Input: dimensioned drawing with shaded views. Units: mm. Origin: part minimum x, y, z. Give positions to 0.01 mm unless a question says otherwise; leave off trailing zeros. Write each loop counter-clockwise with the first axis right and the second up, starting at its lowest first coordinate (ties: lowest second). Pieces come first, ordered by that corner, then holes. Notation, with made-up numbers: (-28.75, 77) -> (1.25, 77) arc R20 cw to (1.25, 109) -> close; hole circle Ø3 at (74.5, -36.75). An arc over 180 degrees is marked (long way). Return JSON: item names as keys, results as strings. Group by question number.
Item 1: Section B-B, the plane z = 0.7. Return loops of the section in (x, y) (1 decimal).
Item 2: Line query: line 1 (Y direction, x = 203.2, z = 1.5); line 2 (Y direction, x = 109.5, z = 1.3) (1 decimal); line 3 (Y direction, x = 114, z = 0.15) (1 decimal). Output: solid intervals per line, ascending. Write a range as [from, to].
Item 3: Section A-A, the plane x = 228.6. Return loops of the section in (y, z).
Item 4: Pin query (flat end, axial travel): P1, Ø4, axis at x = 228.6, y = 152.4, coming from the +Z side. Return the tip coordinate at first contact, or that it passes through.
Item 5: Section D-D, the plane y = 20. Return loops of the section in (x, z).
Item 6: Section C-C, the plane y = 152.4. Return loops of the section in (x, z) (1 decimal).
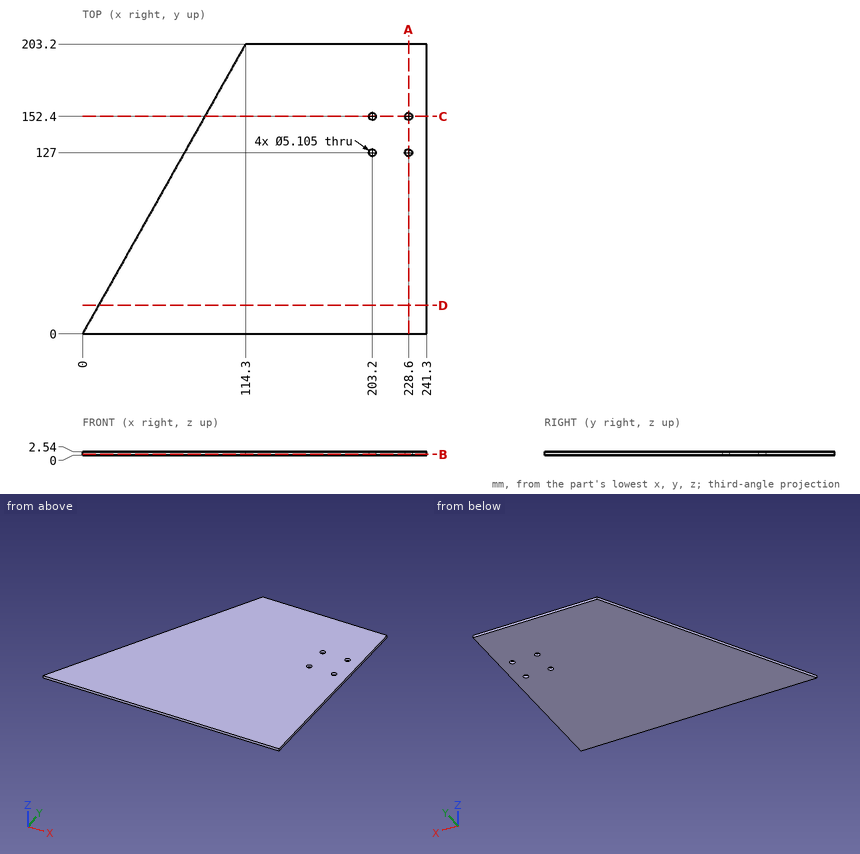
Answer below:
{
 "1": {"outline": "(0, 0) -> (241.3, 0) -> (241.3, 203.2) -> (114.3, 203.2) -> close; hole circle Ø5.1 at (203.2, 127); hole circle Ø5.1 at (203.2, 152.4); hole circle Ø5.1 at (228.6, 127); hole circle Ø5.1 at (228.6, 152.4)"},
 "2": {"line 1": "y = [0, 124.45], [129.55, 149.85], [154.95, 203.2]", "line 2": "y = [0, 194.7]", "line 3": "y = [0, 202.7]"},
 "3": {"outline": "(0, 0) -> (124.45, 0) -> (124.45, 2.54) -> (0, 2.54) -> close; (129.55, 0) -> (149.85, 0) -> (149.85, 2.54) -> (129.55, 2.54) -> close; (154.95, 0) -> (203.2, 0) -> (203.2, 2.54) -> (154.95, 2.54) -> close"},
 "4": {"P1": "passes through"},
 "5": {"outline": "(11.25, 0) -> (241.3, 0) -> (241.3, 2.54) -> (11.25, 2.54) -> close"},
 "6": {"outline": "(85.7, 0) -> (200.6, 0) -> (200.6, 2.5) -> (85.7, 2.5) -> close; (205.8, 0) -> (226, 0) -> (226, 2.5) -> (205.8, 2.5) -> close; (231.2, 0) -> (241.3, 0) -> (241.3, 2.5) -> (231.2, 2.5) -> close"}
}
